Could you check a few things on this drawing? It's one solid part, dimensions in mm from its lowest x, y, z. Coordinates: 2 decimals unless noted, no trailing zeros. Write each loop counter-clockwise with the first axis right and the second up, starting at its lowest first coordinate (ties: lowest second). Pieces come first, ordered by that corner, then holes.
Item 1: I want a section at C-C (y = 2.95). Please give me the cut outline in (x, z), and give its area (3 significant figures).
Item 2: I want a section at D-D (x = 9). Please give me the cut outline in (y, z), and give its area (3 significant figures).
Item 3: Please list where these lines run through material, in increasing order: line 1 (X direction, y = 0.7, z = 40.5); line 2 (X direction, y = 3.5, z = 42.5); line 3 (Z direction, x = 81.5, y = 1.85).
Item 4: I'm going to push a flat-ended pin straight in: P1, Ø6, axis at x = 93, z = 7.5, coming from the +Y side. Where does the tip first touch, or does it pass through?
Item 5: I want a section at A-A (z = 22.5). Please give me the cut outline in (x, y), and give its area (3 significant figures).
Item 6: I want a section at B-B (x = 37.5). Please give me the cut outline in (y, z).
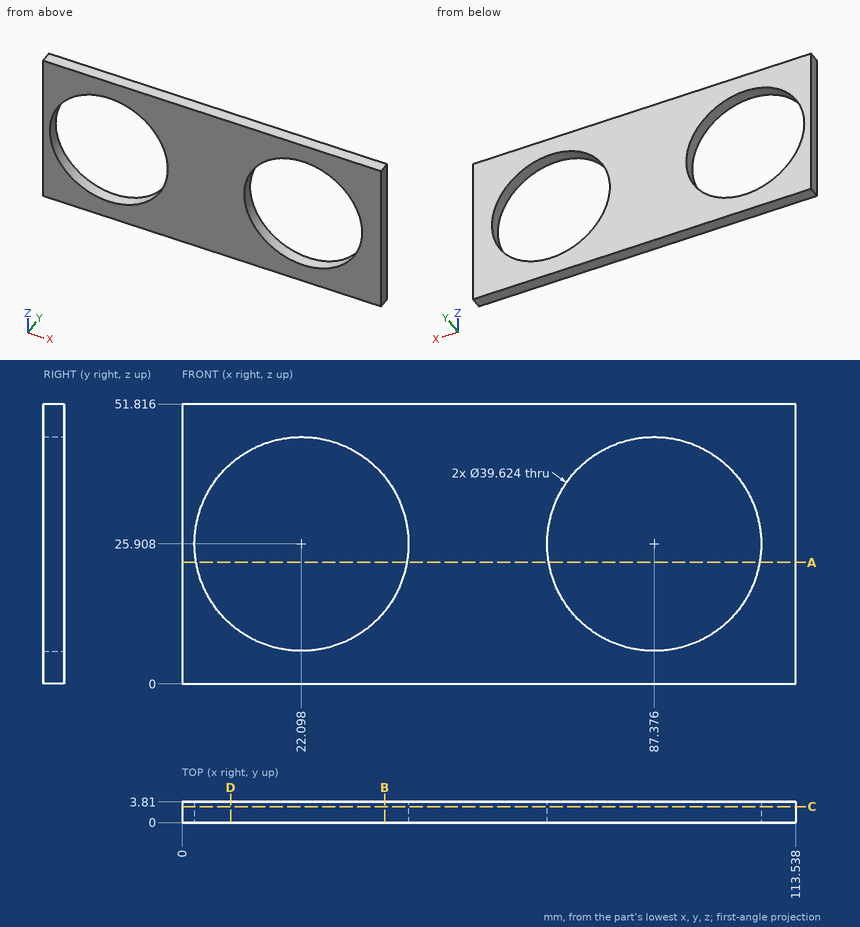
Answer:
1. outline: (0, 0) - (113.54, 0) - (113.54, 51.82) - (0, 51.82) - close; hole circle Ø39.62 at (22.1, 25.91); hole circle Ø39.62 at (87.38, 25.91)
1. area: 3,420 mm2
2. outline: (0, 0) - (3.81, 0) - (3.81, 11.04) - (0, 11.04) - close; (0, 40.77) - (3.81, 40.77) - (3.81, 51.82) - (0, 51.82) - close
2. area: 84.2 mm2
3. line 1: x = 0 to 8.7, 35.5 to 73.97, 100.78 to 113.54
3. line 2: x = 0 to 11.27, 32.92 to 76.55, 98.2 to 113.54
3. line 3: z = 0 to 6.99, 44.83 to 51.82
4. P1: stops at y = 3.81
5. outline: (0, 0) - (2.58, 0) - (2.58, 3.81) - (0, 3.81) - close; (41.61, 0) - (67.86, 0) - (67.86, 3.81) - (41.61, 3.81) - close; (106.89, 0) - (113.54, 0) - (113.54, 3.81) - (106.89, 3.81) - close
5. area: 135 mm2
6. outline: (0, 0) - (3.81, 0) - (3.81, 13.45) - (0, 13.45) - close; (0, 38.37) - (3.81, 38.37) - (3.81, 51.82) - (0, 51.82) - close
